Verification items for the finished model (mm, model axes). Round coordinates to 2 decimals unless told otherwise and drop trailing zeros. Order: outer loops, then holes, each group sorted by start corner. A loop starts at its lowest first (then second) coordinate and runs counter-clockwise, first axis right, second up. Notation, with made-up numbers: (-34.5, -37) -> (-24.5, -37) arc R16 ccw to (-24.5, -22) -> close; hole circle Ø1 at (33, 17). An arc over 180 degrees is marked (long way). Return JSON: item names as keys, results as strings. Group by question number.
1) Scan lines: L1, parallel to Z at x = -0.3, y = 16.4; L2, parallel to Y at x = 0.15, z = 86; L3, parallel to Z at x = 0.2, y = 16. Record each from-to range of solid material in increasing order.
2) Section check D-D on z = -15. Enter the section's corners in (x, y), plus the area to 3 significant figures.
3) Section check A-A on z = 86. Enter the section's corners in (x, y).
4) Depth check by flat-ended pin: pin 1 (5 mm diameter, centred on y = 16.4, z = 78, fed in from +X). Enter the tip coordinate at first touch or a pass-through.
5) Section check C-C on y = 16.4. Enter the section's corners in (x, z).
6) Draft check along Y on faces 1 (the flat face through (-0.5, -5, 1)), 2 (the cylindrical face through (-0.01, 17.37, 87.27)). Enter one of: pulls with the +Y half, pulls with the -Y half, needs draft (parallel to the pull), parting line crosses it, or undercut.
7) Section check B-B on x = 0.1. Enter the section's corners in (y, z), plus the area to 3 significant figures.
Autodesk Inventor part; units mm, degrees
ref_plane "YZ Plane" through (0, 0, 0) normal (1, 0, 0) x (0, 1, 0)
ref_plane "XZ Plane" through (0, 0, 0) normal (0, 1, 0) x (-1, 0, 0)
ref_plane "XY Plane" through (0, 0, 0) normal (0, 0, 1) x (1, 0, 0)
sketch "スケッチ1" plane through (0, 0, 0) normal (1, 0, 0) x (0, 1, 0)
  line L0 (-20.4, 93) -> (20.4, 93)
  line L1 (20.4, 93) -> (20.4, -93)
  line L2 (20.4, -93) -> (-20.4, -93)
  line L3 (-20.4, -93) -> (-20.4, 93)
  line L4 (-20.4, 93) -> (20.4, -93) construction
  line L5 (20.4, 93) -> (-20.4, -93) construction
  point P0 (0, 0)
  dimension "d0" = 40.8
  dimension "d1" = 186
extrude "プレート1" add sketch "スケッチ1" along normal mid plane 1
sketch "スケッチ2" plane through (0.5, 0, 0) normal (1, 0, 0) x (0, 0, -1)
  line L0 (-93, 20.4) -> (93, 20.4)
  line L1 (-93, -20.4) -> (-93, 20.4)
  point P0 (0, 0)
  point P1 (-86, 16.4)
  point P2 (-78, 16.4)
  dimension "d3" = 4
  dimension "d4" = 7
  dimension "d5" = 8
hole "穴1" at (0.5, 16.4, 86) at (0.5, 16.4, 78) direction (-1, 0, 0) diameter 3.2 end through all
sketch "スケッチ3" plane through (-0.5, 0, 0) normal (-1, 0, 0) x (0, 0, 1)
  line L0 (-93, 20.4) -> (-93, -20.4)
  line L1 (-93, 20.4) -> (74, 20.4)
  line L2 (74, 20.4) -> (74, 6.6)
  line L3 (74, 6.6) -> (-93, 6.6)
  line L4 (-93, 6.6) -> (-93, 20.4)
  line L5 (-93, -20.4) -> (93, -20.4)
  line L6 (93, -20.4) -> (93, 20.4)
  point P0 (0, 0)
  point P1 (-93, 6.6)
  dimension "d14" = 19
  dimension "d18" = 13.8
extrude "押し出し1" cut sketch "スケッチ3" against normal blind 10
fillet "コーナーR1" radius 1 4 edges at (0, -20.4, 93) (0, -20.4, -93) (0, 6.6, -93) (0, 6.6, 74)
equation "\"d11\" = Thickness"
equation "\"d2\" = Thickness"
equation "\"BendRadius\" = Thickness"
equation "\"BendReliefWidth\" = Thickness"
equation "\"BendReliefDepth\" = 0.5 * Thickness"
equation "\"CornerReliefSize\" = 4 * Thickness"
equation "\"MinimumRemnant\" = 2 * Thickness"
equation "\"TransitionRadius\" = BendRadius"
equation "\"JacobiRadiusSize\" = BendRadius"
equation "\"GapSize\" = Thickness"
properties part number "s_carbon_plate2" material "CFRP"
Check result:
{
 "1": {"L1": "74 to 76.4, 79.6 to 84.4, 87.6 to 93", "L2": "-20.4 to 14.8, 18 to 20.4", "L3": "74 to 76.45, 79.55 to 84.45, 87.55 to 93"},
 "2": {"outline": "(-0.5, -20.4) -> (0.5, -20.4) -> (0.5, 6.6) -> (-0.5, 6.6) -> close", "area": "27.0 mm^2"},
 "3": {"outline": "(-0.5, -20.4) -> (0.5, -20.4) -> (0.5, 14.8) -> (-0.5, 14.8) -> close; (-0.5, 18) -> (0.5, 18) -> (0.5, 20.4) -> (-0.5, 20.4) -> close"},
 "4": {"pin 1": "x = 0.5"},
 "5": {"outline": "(-0.5, 74) -> (0.5, 74) -> (0.5, 76.4) -> (-0.5, 76.4) -> close; (-0.5, 79.6) -> (0.5, 79.6) -> (0.5, 84.4) -> (-0.5, 84.4) -> close; (-0.5, 87.6) -> (0.5, 87.6) -> (0.5, 93) -> (-0.5, 93) -> close"},
 "6": {"face 1": "needs draft", "face 2": "undercut"},
 "7": {"outline": "(-20.4, -92) arc R1 ccw to (-19.4, -93) -> (5.6, -93) arc R1 ccw to (6.6, -92) -> (6.6, 73) arc R1 cw to (7.6, 74) -> (20.4, 74) -> (20.4, 93) -> (-19.4, 93) arc R1 ccw to (-20.4, 92) -> close; hole circle Ø3.2 at (16.4, 78); hole circle Ø3.2 at (16.4, 86)", "area": "5,270 mm^2"}
}
